Geometry check sheet. Reference: the model listing, model coordinates, mm. Round coordinates to 2 decimals unless told otherwise and drop trailing zeros. Use a Markdown table: item, result. Add a question column.
Item 1: Mould release check, pull along Y, two halves, no side actions. Record for faces 1 (the flat face through (1889, -37.858, 0)), 2 (the flat face through (1540, -44.38, 0)), 3 (the flat face through (1546.518, -49, 0)): pulls with the +Y half, pulls with the -Y half, needs draft (parallel to the pull), parting line crosses it, or undercut.
Item 2: Gauge pin test, flat ends, axial feed: pin 1 Ø2 at (x, z) = (1839.5, -2) entering from -Y; pin 2 Ø3 at (x, z) = (1541, -1.5) entering from -Y; pin 3 Ø1 at (y, z) = (-31, 2) entering from +X. Record the tip position at first contact, or that the pin passes through.
Item 3: Material ranges on probe 1 along X at (y, z) = (-44.5, -1); probe 2 along Y at (x, z) = (1562.5, -0.75); probe 3 along Y at (x, z) = (1710, -2.5), recorded low to high. Write a range as [from, to].
from build123d import *

# Parameters (mm, degrees)
BOSS_EXTRUDE1_DEPTH = 3.175
CUT_EXTRUDE1_DEPTH  = 7.3500001
FILLET1_R           = 2.54
CUT_EXTRUDE2_DEPTH  = 7.62


with BuildPart() as part:
    # Sketch1 → Boss-Extrude1 (new body, symmetric)
    with BuildSketch(Plane.XY):
        with BuildLine():
            Line((499.61002795, -53.470702797), (1046.28548189, -53.470702797))
            add(Edge.make_bspline(
                [(2669.54, -9.569049356), (2615.393603553, -13.17073937), (2561.080658619, -16.536108081), (2506.205230446, -19.758621957), (2430.209106802, -23.505211705), (2354.212983157, -26.631486423), (2332.570330468, -27.480988169), (2156.268639429, -34.377768543), (1979.966947376, -41.628631248), (1824.114277635, -52.771265877), (1636.928606778, -53.579569849), (1449.742935921, -53.454024613), (1418.006730935, -53.470702797), (1324.899336146, -53.470702797), (1231.791940344, -53.470702797), (1170.441269319, -53.470702797), (1108.784075813, -53.470702797), (1047.126882346, -53.470702797), (1046.846414188, -53.470702797), (1046.565947184, -53.470702797), (1046.28548189, -53.470702797)],
                knots=[103.698913506, 103.698913506, 103.698913506, 103.698913506, 103.698913506, 103.698913506, 130.927896619, 130.927896619, 130.927896619, 141.337054719, 141.337054719, 141.337054719, 218.101815019, 218.101815019, 218.101815019, 233.772059419, 233.772059419, 233.772059419, 264.077723219, 264.077723219, 264.077723219, 264.2162088, 264.2162088, 264.2162088, 264.2162088, 264.2162088, 264.2162088], degree=5))
            Line((2669.54, -9.569049356), (2669.54, 9.5231025))
            add(Edge.make_bspline(
                [(2669.54, 9.5231025), (2667.126494524, 9.36235515), (2659.861586685, 8.880281494), (2635.666282302, 7.292469146), (2596.857665529, 4.826056853), (2545.729743039, 1.758344093), (2494.405305707, -1.098555235), (2451.533022267, -3.266573297), (2417.198316756, -4.86708361), (2391.457076919, -6.003589235), (2365.634736307, -7.086854581), (2339.546284672, -8.137729944), (2313.466132974, -9.165138371), (2287.612375486, -10.179478215), (2261.763347437, -11.201032297), (2227.285329715, -12.583842557), (2184.175569393, -14.36607236), (2132.429066114, -16.607427868), (2063.4255234, -19.708920485), (1977.174907635, -23.700543313), (1873.732451432, -28.149389221), (1770.37461881, -31.657468649), (1667.085687813, -33.793117556), (1581.011094491, -34.383188831), (1512.07397126, -34.4278026), (1443.061513477, -34.409510402), (1356.800927879, -34.424432812), (1218.794626954, -34.418464788), (1115.289022786, -34.420702797), (1046.28548189, -34.420702797)],
                knots=[103.571582669, 103.571582669, 103.571582669, 103.571582669, 104.300777207, 105.766098403, 110.877392287, 115.98868617, 121.099980054, 126.211273938, 128.76692088, 131.322567822, 133.878214764, 136.433861706, 138.989508647, 141.545155589, 144.100802531, 146.656449473, 151.767743357, 156.879037241, 161.990331124, 172.212918892, 182.43550666, 192.658094427, 202.880682195, 213.103269962, 218.214563846, 223.32585773, 233.548445497, 243.771033265, 264.2162088, 264.2162088, 264.2162088, 264.2162088], degree=3))
            Line((1046.28548189, -34.420702797), (499.61002795, -34.420702797))
            add(Edge.make_bspline(
                [(499.61002795, -34.420702797), (488.614737518, -34.420702797), (472.236395365, -34.420702798), (449.940231846, -34.420702794), (427.771305695, -34.42070281), (405.874681663, -34.420702712), (384.584909128, -34.420702942), (368.900229326, -34.420702244), (353.376568613, -34.420704862), (332.608466435, -34.420689186), (306.287754853, -34.420570006), (274.023487704, -34.420538256), (252.271015965, -34.420709741), (241.425150134, -34.420702761)],
                knots=[19.90682951, 19.90682951, 19.90682951, 19.90682951, 23.220120017, 24.876765271, 26.533410525, 29.846701033, 31.503346286, 33.15999154, 34.816636794, 36.473282048, 39.786572556, 43.099863063, 46.413153571, 46.413153571, 46.413153571, 46.413153571], degree=3))
            add(Edge.make_bspline(
                [(241.425150134, -34.420702761), (239.394928853, -34.420701455), (235.322322927, -34.420495867), (227.274423443, -34.398702533), (217.319360062, -34.297466855), (205.530690077, -33.976385563), (189.963341914, -33.212641271), (170.696984653, -31.543495194), (147.533261232, -28.314398128), (125.482753206, -24.202109872), (109.358914834, -20.622537553), (100.964116069, -18.612521054), (99.06, -18.149327722)],
                knots=[0, 0, 0, 0, 0.622088422, 1.244176844, 2.488353689, 3.732530533, 4.976707377, 7.465061066, 9.953414755, 12.441768444, 14.55823542, 15.180323842, 15.180323842, 15.180323842, 15.180323842], degree=3))
            Line((99.06, -18.149327722), (99.06, -37.741485304))
            add(Edge.make_bspline(
                [(241.425137875, -53.470702761), (224.286916993, -53.470691732), (207.149474967, -53.467315374), (190.203897513, -52.686577078), (161.734965878, -49.987457476), (133.266034188, -45.175583375), (121.749620566, -42.910592695), (110.349390726, -40.420274627), (99.06, -37.741485304)],
                knots=[0, 0, 0, 0, 0, 0, 8.71381608, 8.71381608, 8.71381608, 14.701907176, 14.701907176, 14.701907176, 14.701907176, 14.701907176, 14.701907176], degree=5))
            add(Edge.make_bspline(
                [(499.61002795, -53.470702797), (492.136820835, -53.470702797), (484.754348064, -53.470702797), (477.443025859, -53.470702797), (448.516583145, -53.470702797), (419.590140517, -53.470702797), (398.368118521, -53.470702797), (355.647540186, -53.470702797), (312.926961851, -53.470702797), (289.235090436, -53.470293029), (265.364963651, -53.470705034), (241.4948369, -53.470702789), (241.471603891, -53.470702785), (241.448370882, -53.470702776), (241.425137875, -53.470702761)],
                knots=[19.90682951, 19.90682951, 19.90682951, 19.90682951, 19.90682951, 19.90682951, 23.637897311, 23.637897311, 23.637897311, 34.276545571, 34.276545571, 34.276545571, 46.401340901, 46.401340901, 46.401340901, 46.413153571, 46.413153571, 46.413153571, 46.413153571, 46.413153571, 46.413153571], degree=5))
        make_face()
    extrude(amount=BOSS_EXTRUDE1_DEPTH, both=True)

    # Sketch2 → Cut-Extrude1 (cut, through all)
    with BuildSketch(Plane.XY.offset(3.175)):
        with BuildLine():
            add(Edge.make_bspline(
                [(2312.9875, -9.183260037), (2304.505441691, -9.516700376), (2287.441020622, -10.186250162), (2261.763347437, -11.201032297), (2228.230552004, -12.545932515), (2203.310445107, -13.575047161), (2187.00995947, -14.263260037)],
                knots=[139.04033329, 139.04033329, 139.04033329, 139.04033329, 141.545155589, 144.100802531, 146.656449473, 151.487488909, 151.487488909, 151.487488909, 151.487488909], degree=3))
            Line((2187.00995947, -14.263260037), (2312.9875, -14.263260037))
            Line((2312.9875, -14.263260037), (2312.9875, -9.183260037))
        make_face()
    extrude(amount=-CUT_EXTRUDE1_DEPTH, mode=Mode.SUBTRACT)

    # Fillet1
    fillet1_edges = [part.edges().sort_by_distance(p)[0] for p in [
        (2669.54, -9.569049356, -1.5875),
        (2669.54, 9.5231025, -1.5875),
        (99.06, -37.741485304, -1.5875),
        (99.06, -18.149327722, -1.5875),
        (2312.9875, -9.183260037, 1.5875),
        (2312.9875, -14.263260037, 0),
    ]]
    fillet(fillet1_edges, radius=FILLET1_R)

    # Sketch3 → Cut-Extrude2 (cut)
    with BuildSketch(Plane.XY.offset(3.175)):
        Polygon((1534.520918045, -34.408934174), (1534.520918045, -44.380222694), (1546.518002564, -44.380222694), (1546.518002564, -53.444776375), (1546.518002564, -106.023211896), (55.693371554, -302.623897547), (0, 180.999666526), (1534.520918045, 89.767095142), align=None)
        Polygon((1888.274985361, -27.424617015), (1881.98614013, -37.858137115), (1895.406326502, -37.858137115), (1895.406326502, -46.204944132), (1895.406326502, -56.664358377), (2711.703422573, -53.444776375), (2711.703422573, 52.291712547), (1888.274985361, 63.130297766), align=None)
    extrude(amount=-CUT_EXTRUDE2_DEPTH, mode=Mode.SUBTRACT)


solid = part.part
Found:
| question | item | result |
|---|---|---|
| 1 | face 1 | undercut |
| 1 | face 2 | pulls with the -Y half |
| 1 | face 3 | needs draft |
| 2 | pin 1 | stops at y = -48.35 |
| 2 | pin 2 | stops at y = -44.38 |
| 2 | pin 3 | stops at x = 1886.42 |
| 3 | probe 1 | x = [1546.52, 1895.41] |
| 3 | probe 2 | y = [-53.41, -34.36] |
| 3 | probe 3 | y = [-51.9, -32.84] |
